Input: part model. Units: mm. Frame: model coordinates. A direction names the side the tool comes from. Coordinates: 2 decimals unless noted, no trailing zeros. Order: outer loops, then holes, each group sorted by start corner. A loop starts at its lowest first (then second) coordinate and runs counter-clockwise, first axis right, second up. Notation, with made-up numbers: (50.25, -30.75) - (103.25, -30.75) arc R19 cw to (103.25, -11.75) - close; hole circle Ø5 at (12, -28). An arc over 180 degrees is marked (long way). Answer as CSV lines item,"result". Start each with the question number.
Item 1: Access query for faces 1 (the cylindrical face through (-5.961, -26.846, 39.049)), 2 (the cylindrical face through (-11.04, 21.87, 11.18)), 3 (the flat face through (-5, 17, 9.3)), 4 (the flat face through (7.922, -29.453, 15.19)). Directions: +Z, -Z, +X, -X, +Y, -Y. A direction counts if a zero-diameter tool reaches every point of the face in a straight line with its end or side. Return the directions, or none.
Item 2: First-contact query: pin 1 (19 mm diameter, centred on x = 0.5, y = 1.5, fed in from -Z); pin 2 (1 mm diameter, centred on y = -8, z = 24.5, fed in from -X); pin 3 (8 mm diameter, centred on y = -26.5, z = 29.5, fed in from +X). Flat tips, straight axial feed; report the tip coordinate or a pass-through.
Item 3: Material intervals for line 1 along Z through (x, y) = (7, -27.5); line 2 along Y through (x, z) = (0, 34.25); line 3 along Z through (x, y) = (26, 11), sorted ascending.
Item 4: Section D-D (z = 5.5). Output: boundary loops of the cut face in (x, y).
Item 5: Section C-C (z = 40.5). Output: boundary loops of the cut face in (x, y).
Item 6: Section B-B (y = -17.5). Output: boundary loops of the cut face in (x, z).
Item 7: Section A-A (z = 28). Output: boundary loops of the cut face in (x, y), and give its area (3 significant figures).
Item 8: Draft query along Z for faces 5 (the cylindrical face through (-21.625, -16.581, 32.065)), 6 (the flat face through (8.578, -31.902, 20.964)), 7 (the cylindrical face through (-2.05, 15.616, 2.218)). Return one class per face: +Z half, -Z half, draft (parallel to the pull), parting line (faces both ways), or undercut.
from build123d import *

# Parameters (mm, degrees)
SKETCH_1_R          = 15.75
EXTRUDE_1_DEPTH     = 4.5
SKETCH_2_R          = 16.3
EXTRUDE_2_DEPTH     = 6
SKETCH_3_R          = 19
EXTRUDE_3_DEPTH     = 0.5
SKETCH_4_R          = 24
EXTRUDE_4_DEPTH     = 0.6
SKETCH_5_R          = 28.5
EXTRUDE_5_DEPTH     = 10
SKETCH_6_R          = 0.8
EXTRUDE_6_DEPTH     = 1.2
SKETCH_7_R          = 29.25
EXTRUDE_7_DEPTH     = 8
SKETCH_8_R          = 27.25
EXTRUDE_8_DEPTH     = 5
SKETCH_9_R          = 28.5
EXTRUDE_9_DEPTH     = 7.9
SKETCH_10_R         = 14.75
CUT_EXTRUDE_1_DEPTH = 1
SKETCH_11_R         = 27.5
CUT_EXTRUDE_2_DEPTH = 7
SKETCH_12_R         = 15
CUT_EXTRUDE_3_DEPTH = 4
EXTRUDE_10_DEPTH    = 0.85
EXTRUDE_START       = 6.75
EXTRUDE_11_DEPTH    = 6.75
EXTRUDE_12_DEPTH    = 8.6
EXTRUDE_16_DEPTH    = 4.2


with BuildPart() as part:
    # 草图1 → 凸台-拉伸1 (new body)
    with BuildSketch(Plane.XY):
        Circle(SKETCH_1_R)
    extrude(amount=EXTRUDE_1_DEPTH)

    # 草图2 → 凸台-拉伸2 (add)
    with BuildSketch(Plane.XY.offset(4.5)):
        Circle(SKETCH_2_R)
    extrude(amount=EXTRUDE_2_DEPTH)

    # 草图3 → 凸台-拉伸3 (add)
    with BuildSketch(Plane.XY.offset(10.5)):
        Circle(SKETCH_3_R)
    extrude(amount=EXTRUDE_3_DEPTH)

    # 草图4 → 凸台-拉伸4 (add)
    with BuildSketch(Plane.XY.offset(11)):
        Circle(SKETCH_4_R)
    extrude(amount=EXTRUDE_4_DEPTH)

    # 草图5 → 凸台-拉伸5 (add)
    with BuildSketch(Plane.XY.offset(11.6)):
        Circle(SKETCH_5_R)
    extrude(amount=EXTRUDE_5_DEPTH)

    # 草图6 → 凸台-拉伸6 (add)
    with BuildSketch(Plane(origin=(0, 0, 10.5), x_dir=(-1, 0, 0), z_dir=(0, 0, -1))):
        with Locations(Location((4.658742812, 17.386664873, 0), (0, 0, 180))):
            Circle(SKETCH_6_R)
    extrude(amount=EXTRUDE_6_DEPTH)

    # 草图7 → 凸台-拉伸7 (add)
    with BuildSketch(Plane.XY.offset(21.6)):
        Circle(SKETCH_7_R)
    extrude(amount=EXTRUDE_7_DEPTH)

    # 草图8 → 凸台-拉伸8 (add)
    with BuildSketch(Plane.XY.offset(29.6)):
        Circle(SKETCH_8_R)
    extrude(amount=EXTRUDE_8_DEPTH)

    # 草图9 → 凸台-拉伸9 (add)
    with BuildSketch(Plane.XY.offset(34.6)):
        Circle(SKETCH_9_R)
    extrude(amount=EXTRUDE_9_DEPTH)

    # 草图10 → 切除-拉伸1 (cut)
    with BuildSketch(Plane(origin=(0, 0, 0), x_dir=(-1, 0, 0), z_dir=(0, 0, -1))):
        Circle(SKETCH_10_R)
    extrude(amount=-CUT_EXTRUDE_1_DEPTH, mode=Mode.SUBTRACT)

    # 草图11 → 切除-拉伸2 (cut)
    with BuildSketch(Plane.XY.offset(42.5)):
        Circle(SKETCH_11_R)
    extrude(amount=-CUT_EXTRUDE_2_DEPTH, mode=Mode.SUBTRACT)

    # 草图12 → 切除-拉伸3 (cut)
    with BuildSketch(Plane.XY.offset(35.5)):
        Circle(SKETCH_12_R)
    extrude(amount=-CUT_EXTRUDE_3_DEPTH, mode=Mode.SUBTRACT)

    # 草图13 → 凸台-拉伸10 (add)
    with BuildSketch(Plane(origin=(0, 0, 11.6), x_dir=(-1, 0, 0), z_dir=(0, 0, -1))):
        with BuildLine():
            Line((6.34130657, 29.833501822), (5.093836425, 23.964616218))
            ThreePointArc((5.093836425, 23.964616218), (11.122767244, 21.829659843), (16.393699856, 18.207048224))
            Line((16.393699856, 18.207048224), (20.408483494, 22.665917177))
            ThreePointArc((20.408483494, 22.665917177), (13.846710242, 27.175698988), (6.34130657, 29.833501822))
        make_face()
    extrude(amount=EXTRUDE_10_DEPTH)

    # 草图14 → 凸台-拉伸11 (add)
    with BuildSketch(Plane.XY.offset(11.6).offset(EXTRUDE_START)):
        with BuildLine():
            Line((-20.408483494, 22.665917177), (-19.739352888, 21.922772352))
            ThreePointArc((-19.739352888, 21.922772352), (-13.392719742, 26.284692464), (-6.133394879, 28.855354222))
            Line((-6.133394879, 28.855354222), (-6.34130657, 29.833501822))
            ThreePointArc((-6.34130657, 29.833501822), (-13.846710242, 27.175698988), (-20.408483494, 22.665917177))
        make_face()
    extrude(amount=-EXTRUDE_11_DEPTH)

    # 草图15 → 凸台-拉伸12 (add)
    with BuildSketch(Plane(origin=(0, 0, 11), x_dir=(-1, 0, 0), z_dir=(0, 0, -1))):
        with BuildLine():
            Line((-8.216276628, -22.549784885), (-9.922425111, -28.917217707))
            Line((-9.922425111, -28.917217707), (-5.86553664, -30.004257697))
            Line((-5.86553664, -30.004257697), (-4.159388158, -23.636824875))
            ThreePointArc((-4.159388158, -23.636824875), (-6.211657082, -23.182219831), (-8.216276628, -22.549784885))
        make_face()
    extrude(amount=-EXTRUDE_12_DEPTH)

    # 草图16 → 凸台-拉伸16 (add)
    with BuildSketch(Plane(origin=(2.028444235, 0.543519995, 0), x_dir=(0, 0, -1), z_dir=(0.9659258262890674, 0.25881904510252446, 0))):
        Polygon((-34.1, -25.25), (-34.1, -35.5), (-22.386751346, -35.5), (-19.5, -30.5), (-19.5, -29.75), (-30.1, -29.75), (-30.1, -25.25), align=None)
    extrude(amount=-EXTRUDE_16_DEPTH)


solid = part.part
Determined:
1,face 1,"+Z"
1,face 2,"-Z"
1,face 3,"-Z, +X, -X, +Y"
1,face 4,"-Z, +X, -Y"
2,pin 1,"stops at z = 1"
2,pin 2,"stops at x = -28.27"
2,pin 3,"stops at x = 18.69"
3,line 1,"z = 11 to 29.6, 30.1 to 34.1, 34.6 to 42.5"
3,line 2,"y = -27.25 to -15, 15 to 27.25"
3,line 3,"z = 11.6 to 29.6, 34.6 to 42.5"
4,outline,"circle Ø32.6 at (0, 0)"
5,outline,"circle Ø57 at (0, 0); hole circle Ø55 at (0, 0)"
6,outline,"(-23.44, 21.6) - (-22.49, 21.6) - (-22.49, 11.6) - (-16.42, 11.6) - (-16.42, 11) - (-7.4, 11) - (-7.4, 10.5) - (7.4, 10.5) - (7.4, 11) - (16.42, 11) - (16.42, 11.6) - (22.49, 11.6) - (22.49, 21.6) - (23.44, 21.6) - (23.44, 29.6) - (20.89, 29.6) - (20.89, 34.6) - (22.49, 34.6) - (22.49, 42.5) - (21.21, 42.5) - (21.21, 35.5) - (-21.21, 35.5) - (-21.21, 42.5) - (-22.49, 42.5) - (-22.49, 34.6) - (-20.89, 34.6) - (-20.89, 29.6) - (-23.44, 29.6) - close"
7,outline,"circle Ø58.5 at (0, 0); (5.67, -29.28) - (7.16, -34.83) - (11.22, -33.75) - (9.73, -28.19) - close"
7,area,"2,710 mm^2"
8,face 5,"undercut"
8,face 6,"-Z half"
8,face 7,"draft"
